Read the model definition and answer for the solid it produces. Units are mm, in the model's axes. A direction names the side the tool comes from. Coordinates: 2 decimals unless noted, no trailing zeros. Loops run counter-clockwise (first coordinate to the right, second up) from the corner with the lowest first, then second, coordinate; pieces in that order, holes last.
Q1. Section B-B (z = 21.9) is taken. Give the vertices of the cut face in (x, y) (3 decimals), then the cut area to 3 significant figures.
Q2. The mould has two halves that part along Y. Classify faces 3 (the face through (-4.769, -21.477, 24.667)), 4 (the face through (-1.5, 0.07, 22.9)), 5 (the face through (0, -5, 24.87)): pulls with the +Y half, pulls with the -Y half, needs draft (parallel to the pull), parting line crosses it, or undercut.
Q3. Straight lines are drawn through the part: line 1 (Y direction, x = 0, z = 21.7) (3 decimals); line 2 (Z direction, x = 11.5, y = -16); line 3 (Z direction, x = 15.5, y = -15). For each, find the intervals that lie inside material, in ascending order.
Q4. Section C-C (x = 18.5) is taken. Count the separate pieces of the cut face and the enclosed holes in it, then the cut area to 3 significant figures.
Q5. Which of the six approach directions +Z, -Z, +X, -X, +Y, -Y give full straight-line access (tool end or side, diameter ignored) to faces 1 (the face through (17.41, 5.48, 22.77)), 2 (the face through (0.65, -6.99, 22.9))?
Q6. Section A-A (x = 0) is taken. Give the vertices of the cut face in (y, z), then the cut area to 3 significant figures.
Q7. A flat-ended cylindrical pin translates along its axis: P1, Ø2, axis at x = -0.5, z = 22, coming from the +Y side. Find the tip coordinate at first contact, or state that the pin passes through.
from build123d import *

# Parameters (mm, degrees)
SKETCH1_R                = 22
BOSS_EXTRUDE1_DEPTH      = 4
M2_CLEARANCE_HOLE1_D     = 2.4
F_1_0_1_DIAMETER_HOLE1_D = 1
F_3_0_3_DIAMETER_HOLE1_D = 3


# Read off the part's stored shape, not the designer's step: Imported1
with BuildPart() as part:
    # Sketch1 → Boss-Extrude1 (new body)
    with BuildSketch(Plane.XY.offset(20.87)):
        Circle(SKETCH1_R)
    extrude(amount=BOSS_EXTRUDE1_DEPTH)

    # M2 Clearance Hole1 (through all)
    with Locations(Plane(origin=(0, 0, 20.87), x_dir=(-1, 0, 0), z_dir=(0, 0, -1))):
        with Locations((0, 8), (-8, 0), (0, -8), (8, 0)):
            Hole(M2_CLEARANCE_HOLE1_D / 2)

    # Sketch4 → Cut-Revolve5 (revolve, cut)
    with BuildSketch(Plane(origin=(0, 0, 0), x_dir=(0, 0, -1), z_dir=(1, 0, 0)), mode=Mode.PRIVATE) as cut_revolve5_sk:
        Polygon((-21.27, 22), (-24.47, 22), (-22.87, 18), align=None)
    revolve(cut_revolve5_sk.sketch.rotate(Axis((0, 0, 24.47), (0, 0, 1)), 270), axis=Axis((0, 0, 24.47), (0, 0, 1)), mode=Mode.SUBTRACT)

    # Ø1.0 (1) Diameter Hole1 (through all)
    with Locations(Plane.XY.offset(24.87)):
        with Locations((18.5, 0)):
            Hole(F_1_0_1_DIAMETER_HOLE1_D / 2)

    # Ø3.0 (3) Diameter Hole1 (through all)
    with Locations(Plane(origin=(0, 0, 20.87), x_dir=(-1, 0, 0), z_dir=(0, 0, -1))):
        with Locations((0, 0)):
            Hole(F_3_0_3_DIAMETER_HOLE1_D / 2)


solid = part.part
Numbers:
1. outline: circle Ø40.85 at (0, 0); hole circle Ø2.4 at (-8, 0); hole circle Ø3 at (0, 0); hole circle Ø2.4 at (0, -8); hole circle Ø2.4 at (0, 8); hole circle Ø2.4 at (8, 0); hole circle Ø1 at (18.5, 0)
1. area: 1,280 mm2
2. face 3: parting line crosses it
2. face 4: undercut
2. face 5: needs draft
3. line 1: y = -20.925 to -9.2, -6.8 to -1.5, 1.5 to 6.8, 9.2 to 20.925
3. line 2: z = 20.87 to 22.19, 23.55 to 24.87
3. line 3: z = 20.87 to 21.44, 24.3 to 24.87
4. separate pieces: 4
4. enclosed holes: 0
4. area: 59.1 mm2
5. face 1: none
5. face 2: +Z, -Z
6. outline: (-22, 20.87) - (-9.2, 20.87) - (-9.2, 24.87) - (-22, 24.87) - (-22, 24.47) - (-18, 22.87) - (-22, 21.27) - close; (-6.8, 20.87) - (-1.5, 20.87) - (-1.5, 24.87) - (-6.8, 24.87) - close; (1.5, 20.87) - (6.8, 20.87) - (6.8, 24.87) - (1.5, 24.87) - close; (9.2, 20.87) - (22, 20.87) - (22, 21.27) - (18, 22.87) - (22, 24.47) - (22, 24.87) - (9.2, 24.87) - close
6. area: 132 mm2
7. P1: stops at y = 22
